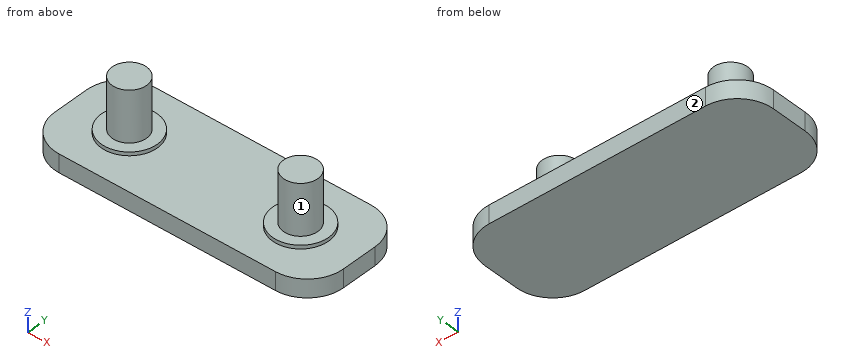
from build123d import *

# Parameters (mm, degrees)
F0_R     = 7.75
F1_DEPTH = 5
F0_R_2   = 4.75
F2_DEPTH = 6
F3_DEPTH = 20


with BuildPart() as f1:
    # F0 (on Top) → F1 (new body)
    with BuildSketch(Plane.XY):
        with BuildLine():
            Line((70, 0), (10, 0))
            ThreePointArc((10, 0), (2.928932, -2.928932), (0, -10))
            Line((0, -10), (0, -20))
            ThreePointArc((0, -20), (2.928932, -27.071068), (10, -30))
            Line((10, -30), (70, -30))
            ThreePointArc((70, -30), (77.071068, -27.071068), (80, -20))
            Line((80, -20), (80, -10))
            ThreePointArc((80, -10), (77.071068, -2.928932), (70, 0))
        make_face()
        with Locations((16.25, -15)):
            Circle(F0_R, mode=Mode.SUBTRACT)
        with Locations((63.75, -15)):
            Circle(F0_R, mode=Mode.SUBTRACT)
    extrude(amount=F1_DEPTH)

    # F0 (on Top) → F2 (join)
    with BuildSketch(Plane.XY):
        with Locations((16.25, -15)):
            Circle(F0_R)
        with Locations((16.25, -15)):
            Circle(F0_R_2, mode=Mode.SUBTRACT)
        with Locations((63.75, -15)):
            Circle(F0_R)
        with Locations((63.75, -15)):
            Circle(F0_R_2, mode=Mode.SUBTRACT)
    extrude(amount=F2_DEPTH)

    # F0 (on Top) → F3 (join)
    with BuildSketch(Plane.XY):
        with Locations((16.25, -15)):
            Circle(F0_R_2)
        with Locations((63.75, -15)):
            Circle(F0_R_2)
    extrude(amount=F3_DEPTH)


solid = f1.part
Check sheet for the modelled part. Datum: model origin and axes. Units: mm. Face numbers are marked on the shaded views. A direction names the side the tool comes from. Coordinates: 2 decimals unless noted, no trailing zeros. Loops run counter-clockwise (first coordinate to the right, second up) from the corner with the lowest first, then second, coordinate; pieces in that order, holes last. Notation, with made-up numbers: (75, 89.5) -> (79, 89.5) arc R17 cw to (79, 113.5) -> close; hole circle Ø2 at (13, 50). An arc over 180 degrees is marked (long way). Answer in a Markdown table with one row per item.
1. Access from +Z, -Z, +X, -X, +Y, -Y to the whole of each face (thin tool, end or side, straight path). Record for the marked faces 1 and 2.
Check values:
| item | result |
|---|---|
| face 1 | +Z |
| face 2 | +Z, -Z, +X, -X, +Y |
2. Sectioned sample at A-A, the plane x = 16.25. Record the boundary of the cut face in (y, z), then the cut area to 4 significant figures.
Check values:
| item | result |
|---|---|
| outline | (-30, 0) -> (0, 0) -> (0, 5) -> (-7.25, 5) -> (-7.25, 6) -> (-10.25, 6) -> (-10.25, 20) -> (-19.75, 20) -> (-19.75, 6) -> (-22.75, 6) -> (-22.75, 5) -> (-30, 5) -> close |
| area | 298.5 mm2 |
3. Sectioned sample at B-B, the plane y = -15. Record the boundary of the cut face in (x, z).
Check values:
| item | result |
|---|---|
| outline | (0, 0) -> (80, 0) -> (80, 5) -> (71.5, 5) -> (71.5, 6) -> (68.5, 6) -> (68.5, 20) -> (59, 20) -> (59, 6) -> (56, 6) -> (56, 5) -> (24, 5) -> (24, 6) -> (21, 6) -> (21, 20) -> (11.5, 20) -> (11.5, 6) -> (8.5, 6) -> (8.5, 5) -> (0, 5) -> close |
4. Sectioned sample at D-D, the plane z = 7.25. Record the boundary of the cut face in (x, y).
Check values:
| item | result |
|---|---|
| outline | circle Ø9.5 at (16.25, -15); circle Ø9.5 at (63.75, -15) |
5. Sectioned sample at C-C, the plane z = 2. Record the boundary of the cut face in (x, y), then the cut area to 3 significant figures.
Check values:
| item | result |
|---|---|
| outline | (0, -20) arc R10 ccw to (10, -30) -> (70, -30) arc R10 ccw to (80, -20) -> (80, -10) arc R10 ccw to (70, 0) -> (10, 0) arc R10 ccw to (0, -10) -> close |
| area | 2,310 mm2 |
6. Go/stop test with flat-tipped pins: pin 1 (3 mm diameter, centred on y = -27, z = 3.5, fed in from -X); pin 2 (4 mm diameter, centred on x = 21, z = 11.5, fed in from -Y); pin 3 (15 mm diameter, centred on x = 50.5, y = -11.5, fed in from +Z). Record where each tip stops, or that it passes through.
Check values:
| item | result |
|---|---|
| pin 1 | stops at x = 1.65 |
| pin 2 | stops at y = -18.87 |
| pin 3 | stops at z = 6 |
7. Material ranges on line 1 along Z through (x, y) = (73.5, -8.5); line 2 along Y through (x, z) = (64, 7.5); line 3 along Z through (x, y) = (22, -12.5), recorded low to high. Write a range as [from, to].
Check values:
| item | result |
|---|---|
| line 1 | z = [0, 5] |
| line 2 | y = [-19.74, -10.26] |
| line 3 | z = [0, 6] |
